For this review, take the finished solid that the model builds, in its own axes (mm). Give positions to 0.01 mm unless a question says otherwise; leave off trailing zeros. Order: outer loops, then holes, each group sorted by start corner. A loop starts at its lowest first (then second) coordinate and runs counter-clockwise, first axis right, second up. Notation, with made-up numbers: (65.5, -21) - (94.5, -21) arc R25 cw to (94.5, -7) - close; hole circle Ø6 at (19, 58.5). An arc over 180 degrees is marked (long way). One line per item, written item: value.
Autodesk Inventor part; units mm, degrees
ref_plane "Work Plane1" through (0, 0, 9.525) normal (0, 0, 1) x (1, 0, 0)
ref_plane "YZ Plane" through (0, 0, 0) normal (1, 0, 0) x (0, 1, 0)
ref_plane "XZ Plane" through (0, 0, 0) normal (0, 1, 0) x (-1, 0, 0)
sketch "Sketch1" plane through (0, 0, 0) normal (0, 0, 1) x (1, 0, 0)
  line L0 (0, 0) -> (0, 15.875)
  line L1 (0, 15.875) -> (0.7937, 15.875)
  line L2 (0.7937, 15.875) -> (0.7938, 0.7937)
  line L3 (0.7938, 0.7937) -> (15.875, 0.7937)
  line L4 (15.875, 0.7937) -> (15.875, 0)
  line L5 (15.875, 0) -> (0, 0)
  dimension "d0" = 15.875
  dimension "d1" = 0.7937
  dimension "d11" = 15.875
extrude "Extrusion1" add sketch "Sketch1" along normal blind 19.05
sketch "Sketch2" plane through (0.7938, 0.7937, 0) normal (1, 0, 0) x (0, 0, -1)
  line L0 (0, 15.0812) -> (0, 0)
  line L1 (-19.05, 0) -> (-19.05, 15.0812)
  circle A0 centre (-9.525, 10.16) radius 1.5875
  line L2 (0, 0) -> (-19.05, 0)
  line L3 (-19.05, 10.16) -> (0, 10.16) construction
  point P0 (0, -0.7937)
  dimension "d4" = 3.175
  dimension "d13" = 10.16
sketch "Sketch3" plane through (0.7938, 0.7937, 0) normal (0, 1, 0) x (1, 0, 0)
  line L0 (15.0812, -19.05) -> (0, -19.05)
  circle A0 centre (10.16, -9.525) radius 1.5875
  line L1 (0, 0) -> (0, -19.05)
  line L2 (10.16, 0) -> (10.16, -19.05) construction
  line L3 (0, 0) -> (15.0812, 0)
  point P0 (-0.7938, 0)
  dimension "d5" = 3.175
  dimension "d10" = 10.16
  dimension "d12" = 15.0813
extrude "Extrusion2" cut sketch "Sketch2" against normal through all
extrude "Extrusion3" cut sketch "Sketch3" against normal through all
ref_plane "Work Plane1" through (0, 0, 9.525) normal (0, 0, 1) x (1, 0, 0)
properties part number "Hopper Pail Mounting Brace P13" material "Aluminum 6061"
(1) For P1, Ø4.5, axis at x = 9, z = 6.5, coming from the +Y side; P2, Ø8, axis at x = 6, y = 5, coming from the -Z side; P3, Ø3.5, axis at x = 10.95, z = 9.52, coming from the -Y side, all flat-tipped, find the tip position at first contact; note any pin that passes through.
Answers below:
P1: stops at y = 0.79
P2: passes through
P3: stops at y = 0
(2) Take a section at C-C (y = 11.25). Write out the cut boundary in (x, z).
Answers below:
outline: (0, 0) - (0.79, 0) - (0.79, 7.97) - (0, 7.97) - close; (0, 11.08) - (0.79, 11.08) - (0.79, 19.05) - (0, 19.05) - close
(3) Wall thickness on line 1 (Y direction, x = 15, z = 8.25): over which ranges is the line inside the solid? List them lowest first. Write a range as from..to.
Answers below:
line 1: y = 0..0.79
(4) Take a section at D-D (z = 10.75). Write out the cut boundary in (x, y) (3 decimals), then the cut area to 3 significant figures.
Answers below:
outline: (0, 0) - (9.944, 0) - (9.944, 0.794) - (0.794, 0.794) - (0.794, 9.944) - (0, 9.944) - close; (0, 11.963) - (0.794, 11.963) - (0.794, 15.875) - (0, 15.875) - close; (11.964, 0) - (15.875, 0) - (15.875, 0.794) - (11.964, 0.794) - close
area: 21.4 mm^2
(5) Take a section at B-B (x = 11). Write out the cut boundary in (y, z).
Answers below:
outline: (0, 0) - (0.79, 0) - (0.79, 7.94) - (0, 7.94) - close; (0, 11.11) - (0.79, 11.11) - (0.79, 19.05) - (0, 19.05) - close
(6) Take a section at A-A (z = 8.25). Write out the cut boundary in (x, y) (1 decimal).
Answers below:
outline: (0, 0) - (10, 0) - (10, 0.8) - (0.8, 0.8) - (0.8, 10) - (0, 10) - close; (0, 11.9) - (0.8, 11.9) - (0.8, 15.9) - (0, 15.9) - close; (11.9, 0) - (15.9, 0) - (15.9, 0.8) - (11.9, 0.8) - close
(7) Draft analysis for pull direction X (two halves, no side actions). For faces 1 (the face through (9.7, 0.4, 10.5)), 2 (the face through (8, 0.794, 9)), 3 (the face through (0, 8, 9)), state which applies: pulls with the +X half, pulls with the -X half, needs draft (parallel to the pull), parting line crosses it, or undercut.
Answers below:
face 1: undercut
face 2: needs draft
face 3: pulls with the -X half
